CAD build for the part. Positions are in the model's coordinates, mm. A direction names the side the tool comes from. Coordinates: 2 decimals unless noted, no trailing zeros. Order: outer loops, then holes, each group sorted by start corner. A loop starts at its lowest first (then second) coordinate and runs counter-clockwise, first axis right, second up. Notation, with made-up numbers: M 20.25,69 L 50.25,69 A13 cw 50.25,91 Z; hole C -26,-19 d8. An arc over 180 degrees is marked long. Write item = value, one per line.
from build123d import *

# Parameters (mm, degrees)
F0_W          = 12
F0_H          = 6
F1_DEPTH      = 4
F3_DEPTH      = 2
F4_W          = 1
F4_H          = 1.2
F4_H_2        = 0.4
F5_DEPTH      = 1
F5_DEPTH_BACK = 0.4


with BuildPart() as f1:
    # F0 (on Top) → F1 (new body)
    with BuildSketch(Plane.XY):
        with Locations((6, 0)):
            Rectangle(F0_W, F0_H)
    extrude(amount=F1_DEPTH)

    # F2 (on face) → F3 (join)
    with BuildSketch(Plane(origin=(0, 0, 0), x_dir=(0, -1, 0), z_dir=(-1, 0, 0))):
        with BuildLine():
            ThreePointArc((1.8874586088, 0), (2.5251743677, 0.910966294), (2.75, 2))
            ThreePointArc((2.75, 2), (2.5251743677, 3.089033706), (1.8874586088, 4))
            Line((1.8874586088, 4), (-1.8874586088, 4))
            ThreePointArc((-1.8874586088, 4), (-2.75, 2), (-1.8874586088, 0))
            Line((-1.8874586088, 0), (1.8874586088, 0))
        make_face()
        with BuildLine():
            Line((-1.8874586088, 4), (1.8874586088, 4))
            ThreePointArc((1.8874586088, 4), (0, 4.75), (-1.8874586088, 4))
        make_face()
        with BuildLine():
            ThreePointArc((-1.8874586088, 0), (0, -0.75), (1.8874586088, 0))
            Line((1.8874586088, 0), (-1.8874586088, 0))
        make_face()
    extrude(amount=F3_DEPTH)

    # F4 (on face) → F5 (join, two sides)
    with BuildSketch(Plane(origin=(0, 0, 0), x_dir=(1, 0, 0), z_dir=(0, 0, -1))) as f5_sk:
        with Locations((1.6, -3.6)):
            Rectangle(F4_W, F4_H)
        with Locations((1.6, 3.6)):
            Rectangle(F4_W, F4_H)
        with Locations((1.6, 2.8)):
            Rectangle(F4_W, F4_H_2)
        with Locations((5.35, 2.8)):
            Rectangle(F4_W, F4_H_2)
        with Locations((5.35, 3.6)):
            Rectangle(F4_W, F4_H)
        with Locations((1.6, -2.8)):
            Rectangle(F4_W, F4_H_2)
        with Locations((5.35, -3.6)):
            Rectangle(F4_W, F4_H)
        with Locations((5.35, -2.8)):
            Rectangle(F4_W, F4_H_2)
        with Locations((9.9, 2.8)):
            Rectangle(F4_W, F4_H_2)
        with Locations((9.9, 3.6)):
            Rectangle(F4_W, F4_H)
    extrude(amount=F5_DEPTH)
    extrude(f5_sk.sketch, amount=-F5_DEPTH_BACK)


solid = f1.part
(1) Pull direction X, two halves, no side cores. Call faces 1 (the face through (2.1, -3.4, -0.3)), 2 (the face through (5, 4, 0.4)), 3 (the face through (5.85, -3.4, -0.3)), 4 (the face through (12, 0, 2)): +X half, -X half, draft (parallel to the pull), parting line (faces both ways), or undercut.
Evaluation:
face_1 = undercut
face_2 = draft
face_3 = undercut
face_4 = +X half
(2) Slice it at B-B, the plane y = -3.5. Write the cut outline in (x, z), then the cut area to 3 significant figures.
Evaluation:
outline = M 1.1,-1 L 2.1,-1 L 2.1,0.4 L 1.1,0.4 Z; M 4.85,-1 L 5.85,-1 L 5.85,0.4 L 4.85,0.4 Z; M 9.4,-1 L 10.4,-1 L 10.4,0.4 L 9.4,0.4 Z
area = 4.20 mm²
(3) Slice it at A-A, the plane z = -0.2. Write the cut outline in (x, y).
Evaluation:
outline = M -2,-1.65 L 0,-1.65 L 0,1.65 L -2,1.65 Z; M 1.1,-4.2 L 2.1,-4.2 L 2.1,-2.6 L 1.1,-2.6 Z; M 1.1,2.6 L 2.1,2.6 L 2.1,4.2 L 1.1,4.2 Z; M 4.85,-4.2 L 5.85,-4.2 L 5.85,-2.6 L 4.85,-2.6 Z; M 4.85,2.6 L 5.85,2.6 L 5.85,4.2 L 4.85,4.2 Z; M 9.4,-4.2 L 10.4,-4.2 L 10.4,-2.6 L 9.4,-2.6 Z
(4) Tool access for faces 5 (the face through (10, -4, 0.4)), 6 (the face through (9.4, -3.4, -0.3)), 7 (the face through (1.6, 3.6, 0.4)), 8 (the face through (2.1, 3.4, -0.3)), 9 (the face through (6, 0, 4)): list every direction of +Z, -Z, +X, -X, +Y, -Y with a clear straight run to the whole face (end or side of a thin tool).
Evaluation:
face_5 = +Z, +X, -X, -Y
face_6 = -Z, -Y
face_7 = +Z, +X, -X, +Y
face_8 = -Z, +Y
face_9 = +Z, +X, +Y, -Y
(5) Pin check, flat tips, straight feed: pin 1 Ø1.5 at (x, y) = (6.5, -1.5) entering from +Z; pin 2 Ø0.7 at (y, z) = (3.5, -0.5) entering from -X; pin 3 Ø1.8 at (x, y) = (7, -1) entering from -Z; pin 4 Ø1 at (y, z) = (-2, 0) entering from -X. Stop position of each tip, or through.
Evaluation:
pin_1 = 4
pin_2 = 1.1
pin_3 = 0
pin_4 = -2
(6) Slice it at D-D, the plane y = -0.75. Write the cut outline in (x, z), then the cut area to 3 significant figures.
Evaluation:
outline = M -2,-0.65 L 0,-0.65 L 0,0 L 12,0 L 12,4 L 0,4 L 0,4.65 L -2,4.65 Z
area = 58.6 mm²
(7) Wall check: line 1 (Z direction, x = 10.5, y = 2); line 2 (Y direction, x = 5, z = 2.3); line 3 (X direction, y = 0, z = -0.6). Give the ranges that are in metal, low to high. Write a range as from..to.
Evaluation:
line_1 = 0..4
line_2 = -3..3
line_3 = -2..0
(8) Slice it at C-C, the plane x = 1.75. Write the cut outline in (y, z), then the cut area to 3 significant figures.
Evaluation:
outline = M -4.2,-1 L -2.6,-1 L -2.6,0 L 2.6,0 L 2.6,-1 L 4.2,-1 L 4.2,0.4 L 3,0.4 L 3,4 L -3,4 L -3,0.4 L -4.2,0.4 Z
area = 28.2 mm²
